Print and shaded views of the part. All mm, measured from the part's lowest x, y and z. Round coordinates to 2 decimals unless told otherwise and drop trailing zeros. Write each loop counter-clockwise with the first axis right and the second up, starting at its lowest first coordinate (ties: lowest second). Pieces come first, ordered by that corner, then holes. Notation, with made-up numbers: (33.5, 82.5) - (50.5, 82.5) arc R27 cw to (50.5, 118.5) - close; hole circle Ø1 at (-18, 8.25). An arc over 180 degrees is marked (long way). One line per item, written item: value.
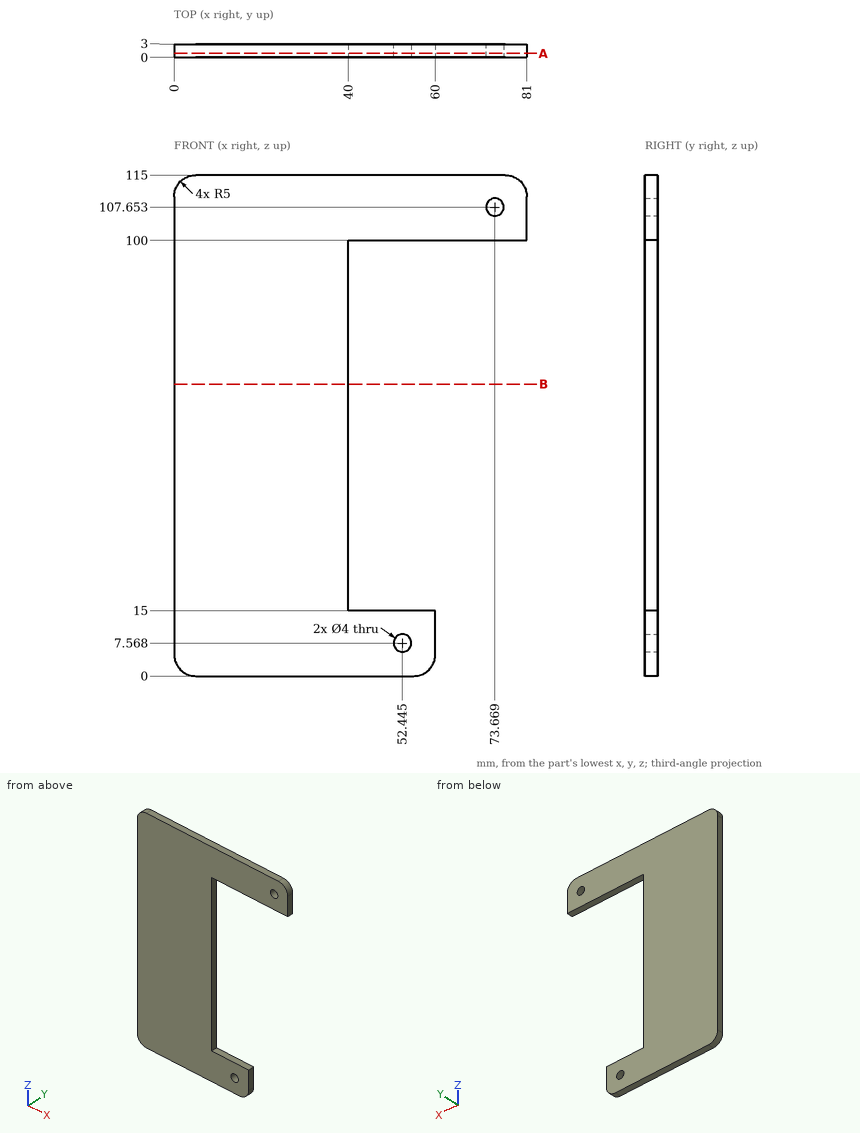
1. Band-saw the part on A-A on y = 0.85. Write the cut outline in (x, z) (1 decimal).
Report:
outline: (0, 5) arc R5 ccw to (5, 0) - (55, 0) arc R5 ccw to (60, 5) - (60, 15) - (40, 15) - (40, 100) - (81, 100) - (81, 110) arc R5 ccw to (76, 115) - (5, 115) arc R5 ccw to (0, 110) - close; hole circle Ø4 at (52.4, 7.6); hole circle Ø4 at (73.7, 107.7)
2. Band-saw the part on B-B on z = 67. Write the cut outline in (x, y).
Report:
outline: (0, 0) - (40, 0) - (40, 3) - (0, 3) - close
3. Wall check: probe 1 along Z at (x, y) = (48, 2.4); probe 2 along Z at (x, y) = (52, 2.55); probe 3 along X at (y, z) = (1.65, 53.5). Give the ranges that are in metal, low to high. Write a range as [from, to].
Report:
probe 1: [0, 15], [100, 115]
probe 2: [0, 5.62], [9.52, 15], [100, 115]
probe 3: [0, 40]
4. Drop flat-ended pins along their axis: pin 1 (1.5 mm diameter, centred on y = 2, z = 70.5, fed in from +X); pin 2 (3.5 mm diameter, centred on x = 52.45, z = 7.57, fed in from +Y); pin 3 (0.9 mm diameter, centred on x = 69, y = 1, fed in from -Z); pin 4 (1.5 mm diameter, centred on y = 1.5, z = 7.5, fed in from +X). Give the stop position or say it passes through.
Report:
pin 1: x = 40
pin 2: through
pin 3: z = 100
pin 4: x = 60
